Autodesk Inventor part; units mm, degrees
ref_plane "YZ Plane" through (0, 0, 0) normal (1, 0, 0) x (0, 1, 0)
ref_plane "XZ Plane" through (0, 0, 0) normal (0, 1, 0) x (-1, 0, 0)
ref_plane "XY Plane" through (0, 0, 0) normal (0, 0, 1) x (1, 0, 0)
sketch "スケッチ1" plane through (0, 0, 0) normal (0, 0, 1) x (1, 0, 0)
  circle A0 centre (-10.9779, 15.759) radius 1.5
  circle A1 centre (-12.7279, 12.7279) radius 1.25
  circle A2 centre (-16.2279, 12.7279) radius 1.5
  circle A3 centre (-10.9779, 9.6968) radius 1.5
  circle A4 centre (-12.7279, 12.7279) radius 6
  circle A5 centre (0, 0) radius 4
  circle A6 centre (0, 0) radius 1.25
  arc A7 (3.9022, 0.8792) -> (-10.2779, 18.2049) centre (-20.4864, -4.6158) ccw
  arc A8 (-18.2049, 10.2779) -> (-0.8792, -3.9022) centre (4.6158, 20.4864) ccw
  circle A9 centre (-12.7279, 12.7279) radius 1.5
  circle A10 centre (-16.2279, 12.7279) radius 1.5
  circle A11 centre (-12.7279, 12.7279) radius 1.25
  circle A12 centre (-10.9779, 9.6968) radius 1.5
  circle A13 centre (-10.9779, 15.759) radius 1.5
  circle A14 centre (-12.7279, 12.7279) radius 6
  circle A15 centre (0, 0) radius 4
  circle A16 centre (0, 0) radius 1.25
  arc A17 (3.9022, 0.8792) -> (-10.2779, 18.2049) centre (-20.4864, -4.6158) ccw
  arc A18 (-18.2049, 10.2779) -> (-0.8792, -3.9022) centre (4.6158, 20.4864) ccw
  circle A19 centre (-12.7279, 12.7279) radius 1.5
  dimension "d0" = 8
  dimension "d1" = 2.5
  dimension "d2" = 25
  dimension "d3" = 3
  dimension "d6" = 8
  dimension "d7" = 2.5
  dimension "d8" = 25
  dimension "d9" = 3
  dimension "d19" = 3
  dimension "d20" = 2.5
extrude "押し出し1" add sketch "スケッチ1" along normal blind 3 contours A4 | A4 A7 A5 A8 | A5
sketch "スケッチ2" plane through (0, 0, 3) normal (0, 0, 1) x (1, 0, 0)
  circle A0 centre (-12.7279, 12.7279) radius 1.5
  circle A1 centre (-12.7279, 12.7279) radius 4
  point P0 (0, 0)
  dimension "d10" = 8
extrude "押し出し2" cut sketch "スケッチ2" against normal blind 0.8
sketch "スケッチ3" plane through (0, 0, 0) normal (0, 0, -1) x (-1, 0, 0)
  circle A0 centre (12.7279, 12.7279) radius 1.5
  circle A1 centre (12.7279, 12.7279) radius 10
  arc A2 (0.8792, -3.9022) -> (18.2049, 10.2779) centre (-4.6158, 20.4864) ccw
  arc A3 (18.2049, 10.2779) -> (10.2779, 18.2049) centre (12.7279, 12.7279) ccw
  arc A4 (10.2779, 18.2049) -> (-3.9022, 0.8792) centre (20.4864, -4.6158) ccw
  arc A5 (-3.9022, 0.8792) -> (0.8792, -3.9022) centre (0, 0) ccw
  circle A6 centre (0, 0) radius 1.25
  circle A7 centre (16.2279, 12.7279) radius 1.5
  circle A8 centre (12.7279, 12.7279) radius 1.5
  circle A9 centre (10.9779, 9.6968) radius 1.5
  circle A10 centre (10.9779, 15.759) radius 1.5
  point P0 (12.9839, 2.7312)
  point P1 (2.7312, 12.9839)
  dimension "d13" = 20
extrude "押し出し3" add sketch "スケッチ3" against normal blind 1.5 contours A1 A2 A3 A4 picked at (8.342, 18.6804)
equation "\"d1\" = d20"
equation "\"d3\" = d9"
equation "\"d7\" = d1"
equation "\"d9\" = d19"
properties part number "原動節4" material "アルミニウム 2014-T4"
Part model, mm, in its own coordinate system. A direction names the side the tool comes from. Coordinates: 2 decimals unless noted, no trailing zeros. Loops run counter-clockwise (first coordinate to the right, second up) from the corner with the lowest first, then second, coordinate; pieces in that order, holes last. Notation, with made-up numbers: (-15, -37) - (34, -37) arc R17 cw to (34, -6) - close; hole circle Ø5 at (21.5, -24.75). An arc over 180 degrees is marked (long way). Write item = value, one per line. Start each with the question number.
Item 1: Cut at B-B, the plane x = 0. Give the cut face in (y, z).
Item 2: Wall check: L1, parallel to Y at x = -10.25, z = 0.95; L2, parallel to Y at x = -10.5, z = 1.6; L3, parallel to X at y = 12, z = 1.4. Give the ranges that are in metal, low to high. Write a range as from..to.
Item 3: Cut at D-D, the plane x = -19.25. Give the cut face in (y, z), and give its area (3 significant figures).
Item 4: 3-axis set-ups, long thin cutter, end or side, ignore diameter. For faces 1 (the cylindrical face through (0.298, 9.277, 1.812)), 2 (the cylindrical face through (-14.76, 9.283, 2.606)), 3 (the cylindrical face through (-9.005, -0.477, 1.812)): which of +Z, -Z, +X, -X, +Y, -Y reach the whole face in a straight line?
Item 5: Cut at C-C, the plane x = -3.25. Give the cut face in (y, z).
Item 6: Flat gauge pin, fed straight in: pin 1 Ø3.5 at (x, y) = (-12.73, 12.73) entering from +Z. Where does the tip first touch, or does it go through?
Item 7: Cut at A-A, the plane y = 0. Give the cut face in (x, z), and give its area (3 significant figures).
The answers:
q1.outline = (-4, 0) - (-1.25, 0) - (-1.25, 3) - (-4, 3) - close; (1.25, 0) - (9.71, 0) - (9.71, 3) - (1.25, 3) - close
q2.L1 = 0.39..8.39, 11.01..14.45, 17.07..22.42
q2.L2 = 0.57..8.27, 11.12..14.34, 17.18..18.3
q2.L3 = -22.7..-17.54, -14.92..-14.04, -11.42..-1.81
q3.outline = (5.15, 0) - (20.31, 0) - (20.31, 1.5) - (5.15, 1.5) - close
q3.area = 22.7 mm2
q4.face_1 = +Z, +X, +Y
q4.face_2 = +Z
q4.face_3 = +Z, -X, -Y
q5.outline = (-3.24, 0) - (15.92, 0) - (15.92, 1.5) - (13.49, 1.5) - (13.49, 3) - (-3.24, 3) - close
q6.pin_1 = 2.2
q7.outline = (-9.71, 0) - (-1.25, 0) - (-1.25, 3) - (-9.71, 3) - close; (1.25, 0) - (4, 0) - (4, 3) - (1.25, 3) - close
q7.area = 33.6 mm2
